Geometry check sheet. Reference: the model listing, model coordinates, mm. A direction names the side the tool comes from. Give positions to 0.01 mm unless a question says otherwise; leave off trailing zeros. Write each loop counter-clockwise with the first axis right and the second up, starting at its lowest first coordinate (ties: lowest second). Pieces come first, ordered by that corner, then holes. Notation, with made-up numbers: (57, -34.75) -> (87, -34.75) arc R29 ccw to (87, 1.25) -> close; hole circle Ø5 at (54, 24). An arc over 180 degrees is marked (long way). Write item = value, one per line. Start each with the question number.
1. Cross-section at B-B, the plane z = -26.5. Record the cut outline in (x, y).
2. Depth check by flat-ended pin: P1, Ø3, axis at x = -24, z = -13.5, coming from the +Y side; P2, Ø8, axis at x = -21.5, z = 28, coming from the -Y side; P3, Ø2, axis at y = 16, z = 36.5, coming from the -X side. Enter the tip coordinate at first touch or a pass-through.
3. Cross-section at D-D, the plane z = 5. Record the cut outline in (x, y).
4. Set-up check for faces 4 (the flat face through (-30.32, 8.18, 16.75)), 5 (the flat face through (-0.65, 8.18, 34.63)), 6 (the flat face through (14.07, 17.08, 32.37)), 7 (the flat face through (-14.07, 17.08, -32.37)): record each of +Z, -Z, +X, -X, +Y, -Y from which the full face is reachable in a straight line by a thin tool's end or side.
5. Mould release check, pull along Z, two halves, no side actions. Record for faces 1 (the cylindrical face through (-41.62, 9.04, 23.91)), 2 (the cylindrical face through (-41.517, 9.042, -24.089)), 3 (the cylindrical face through (-25, 9, 0)): pulls with the +Z half, pulls with the -Z half, needs draft (parallel to the pull), parting line crosses it, or undercut.
6. Cross-section at C-C, the plane x = 15.5. Record the cut outline in (y, z).
7. Thickness scan on line 1 along Y through (x, z) = (8, 24); line 2 along Y through (x, z) = (12.5, -25); line 3 along Y through (x, z) = (-20, -40). Record the ranges inside material, lowest first.
8. Cross-section at A-A, the plane x = 28.5. Record the cut outline in (y, z), plus the area to 3 significant figures.
```python
from build123d import *

# Parameters (mm, degrees)
SKETCH1_R           = 25
BOSS_EXTRUDE1_DEPTH = 18
BOSS_EXTRUDE2_DEPTH = 38
CIRPATTERN1_COUNT   = 6
SKETCH4_R           = 55.206013126
SKETCH4_R_2         = 48
CUT_EXTRUDE2_DEPTH  = 38


with BuildPart() as part:
    # Sketch1 → Boss-Extrude1 (new body)
    with BuildSketch(Plane(origin=(0, 0, 0), x_dir=(1, 0, 0), z_dir=(0, 1, 0))):
        Circle(SKETCH1_R)
    extrude(amount=BOSS_EXTRUDE1_DEPTH)

    # Sketch3 → Boss-Extrude2 (add)
    with BuildSketch(Plane(origin=(0, 0, 48), x_dir=(-1, 0, 0), z_dir=(0, 0, -1))):
        Polygon((-21.362842742, 1.867051803), (20.645822822, 18), (21.362842742, 16.132948197), (-20.645822822, 0), align=None)
    boss_extrude2 = extrude(amount=BOSS_EXTRUDE2_DEPTH)

    # CirPattern1: Boss-Extrude2 ×6 about axis
    cirpattern1_axis = Axis((0, 0, 0), (0, 1, 0))
    for i in range(1, CIRPATTERN1_COUNT):
        add(boss_extrude2.rotate(cirpattern1_axis, i * 360 / CIRPATTERN1_COUNT))

    # Sketch4 → Cut-Extrude2 (cut)
    with BuildSketch(Plane(origin=(0, 18, 0), x_dir=(1, 0, 0), z_dir=(0, 1, 0))):
        Circle(SKETCH4_R)
        Circle(SKETCH4_R_2, mode=Mode.SUBTRACT)
    extrude(amount=-CUT_EXTRUDE2_DEPTH, mode=Mode.SUBTRACT)


solid = part.part
```
Answers:
q1.outline = (-40.02, 9.06) -> (-3.17, 16.13) -> (-4.61, 18) -> (-40.02, 11.2) -> close; (-21.36, 1.87) -> (-20.65, 0) -> (21.36, 16.13) -> (20.65, 18) -> close; (3.17, 1.87) -> (4.61, 0) -> (40.02, 6.8) -> (40.02, 8.94) -> close
q2.P1 = 10.53
q2.P2 = 1.21
q2.P3 = -21.36
q3.outline = (-47.74, 15.43) -> (-24.49, 10.97) -> (-24.49, 3.7) -> (-34.07, 1.87) -> (-32.63, 0) -> (-24.49, 1.56) -> (-24.49, 0) -> (24.49, 0) -> (24.49, 4.89) -> (47.74, 0.42) -> (47.74, 2.57) -> (24.49, 7.03) -> (24.49, 14.3) -> (34.07, 16.13) -> (32.63, 18) -> (24.49, 16.44) -> (24.49, 18) -> (-24.49, 18) -> (-24.49, 13.11) -> (-47.74, 17.58) -> close
q4.face_4 = -X
q4.face_5 = +Z
q4.face_6 = +Z, +Y
q4.face_7 = -Z, +Y
q5.face_1 = pulls with the +Z half
q5.face_2 = pulls with the -Z half
q5.face_3 = undercut
q6.outline = (0, -32.79) -> (1.87, -33.62) -> (6.52, -19.62) -> (13.88, -19.62) -> (13.88, -45.43) -> (16.02, -45.43) -> (16.02, -19.62) -> (18, -19.62) -> (18, 19.62) -> (13.62, 19.62) -> (18, 32.79) -> (16.13, 33.62) -> (11.48, 19.62) -> (4.12, 19.62) -> (4.12, 45.43) -> (1.98, 45.43) -> (1.98, 19.62) -> (0, 19.62) -> (0, -19.62) -> (4.38, -19.62) -> close
q7.line_1 = 4.86 to 7, 14.37 to 16.52
q7.line_2 = 2.01 to 4.16, 12.73 to 14.87
q7.line_3 = 0.25 to 2.39
q8.outline = (0, -7.39) -> (1.87, -8.21) -> (17.44, 38.62) -> (15.3, 38.62) -> close; (0.56, -38.62) -> (2.7, -38.62) -> (18, 7.39) -> (16.13, 8.21) -> close
q8.area = 199 mm^2
